```python
from build123d import *

# Parameters (mm, degrees)
F0_W     = 58
F0_H     = 58
F0_R     = 18.5
F1_DEPTH = 58
F2_W     = 58
F2_H     = 35
F3_DEPTH = 13
F4_W     = 58
F4_H     = 35
F5_DEPTH = 13
F7_D     = 6.8


with BuildPart() as f1:
    # F0 (on Front) → F1 (new body)
    with BuildSketch(Plane.XZ):
        with Locations((29, 29)):
            Rectangle(F0_W, F0_H)
        with Locations((29, 29)):
            Circle(F0_R, mode=Mode.SUBTRACT)
    extrude(amount=F1_DEPTH)

    # F2 (on face) → F3 (cut)
    with BuildSketch(Plane.XY.offset(58)):
        with Locations((29, -27.5)):
            Rectangle(F2_W, F2_H)
    extrude(amount=-F3_DEPTH, mode=Mode.SUBTRACT)

    # F4 (on face) → F5 (cut)
    with BuildSketch(Plane(origin=(0, 0, 0), x_dir=(1, 0, 0), z_dir=(0, 0, -1))):
        with Locations((29, 27.5)):
            Rectangle(F4_W, F4_H)
    extrude(amount=-F5_DEPTH, mode=Mode.SUBTRACT)

    # F7 (through all)
    with Locations(Plane.XZ.offset(58)):
        with Locations((5.5, 52.5), (52.5, 52.5), (5.5, 5.5), (52.5, 5.5)):
            Hole(F7_D / 2)


solid = f1.part
```
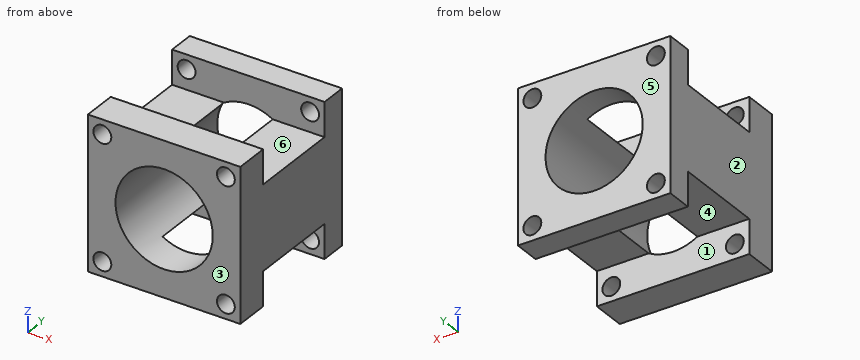
The listing builds one solid part. Answer for the finished solid, in the listing's coordinates (mm). Face numbers are marked on the shaded views. A direction names the side the tool comes from. Give positions to 0.01 mm unless a question says otherwise; leave off trailing zeros. Order: outer loops, then holes, each group sorted by start corner. A loop starts at its lowest first (then second) coordinate and runs counter-clockwise, first axis right, second up.
Item 1: The part is cut by section C-C, the plane z = 29. Give the vertices of the cut face in (x, y).
From the geometry:
outline: (0, -58) - (10.5, -58) - (10.5, 0) - (0, 0) - close; (47.5, -58) - (58, -58) - (58, 0) - (47.5, 0) - close
Item 2: The part is cut by section D-D, the plane y = -49.5. Give the vertices of the cut face in (x, z), and give its area (3 significant figures).
From the geometry:
outline: (0, 0) - (58, 0) - (58, 58) - (0, 58) - close; hole circle Ø6.8 at (5.5, 5.5); hole circle Ø6.8 at (5.5, 52.5); hole circle Ø37 at (29, 29); hole circle Ø6.8 at (52.5, 5.5); hole circle Ø6.8 at (52.5, 52.5)
area: 2,140 mm2
Item 3: Which of the six approach directions +Z, -Z, +X, -X, +Y, -Y give full straight-line access (tool end or side, diameter ignored) to the marked faces 4, 5 and 6?
From the geometry:
face 4: -Z, +X, -X
face 5: +Z, -Z, +X, -X, +Y
face 6: +Z, +X, -X
Item 4: The part is cut by section B-B, the plane x = 5.5. Give the vertices of the cut face in (y, z), and give its area (3 significant figures).
From the geometry:
outline: (-58, 0) - (-45, 0) - (-45, 2.1) - (-58, 2.1) - close; (-58, 8.9) - (-45, 8.9) - (-45, 13) - (-10, 13) - (-10, 8.9) - (0, 8.9) - (0, 49.1) - (-10, 49.1) - (-10, 45) - (-45, 45) - (-45, 49.1) - (-58, 49.1) - close; (-58, 55.9) - (-45, 55.9) - (-45, 58) - (-58, 58) - close; (-10, 0) - (0, 0) - (0, 2.1) - (-10, 2.1) - close; (-10, 55.9) - (0, 55.9) - (0, 58) - (-10, 58) - close
area: 2,140 mm2
Item 5: The part is cut by section A-A, the plane z = 52.5. Give the vertices of the cut face in (x, y).
From the geometry:
outline: (0, -58) - (2.1, -58) - (2.1, -45) - (0, -45) - close; (0, -10) - (2.1, -10) - (2.1, 0) - (0, 0) - close; (8.9, -58) - (49.1, -58) - (49.1, -45) - (8.9, -45) - close; (8.9, -10) - (49.1, -10) - (49.1, 0) - (8.9, 0) - close; (55.9, -58) - (58, -58) - (58, -45) - (55.9, -45) - close; (55.9, -10) - (58, -10) - (58, 0) - (55.9, 0) - close
Item 6: For a pull along Y with two mould halves and no side action, classify the marked faces 1, 2 and 3 as pulls with the +Y half, pulls with the -Y half, needs draft (parallel to the pull), parting line crosses it, or undercut.
From the geometry:
face 1: undercut
face 2: needs draft
face 3: pulls with the -Y half
Item 7: Given pin 1 Ø6 at (x, y) = (46, -26.5) entering from +Z; pin 2 Ø9 at (x, z) = (52.5, 5.5) entering from +Y; pin 3 Ø5.5 at (x, z) = (5.5, 5.5) entering from -Y; pin 4 Ø6 at (x, y) = (52.5, -28) entering from -Z, each flat-ended and moving along its own axis, determine where each tip first touches the part or whether it passes through.
From the geometry:
pin 1: stops at z = 45
pin 2: stops at y = 0
pin 3: passes through
pin 4: stops at z = 13
Item 8: Find the intervals of material crossed by probe 1 along Z at (x, y) = (5.5, -7); probe 2 along Y at (x, z) = (34, 10); probe 3 along X at (y, z) = (-52, 5), in increasing order.
From the geometry:
probe 1: z = 0 to 2.1, 8.9 to 49.1, 55.9 to 58
probe 2: y = -58 to -45, -10 to 0
probe 3: x = 0 to 2.14, 8.86 to 49.14, 55.86 to 58
